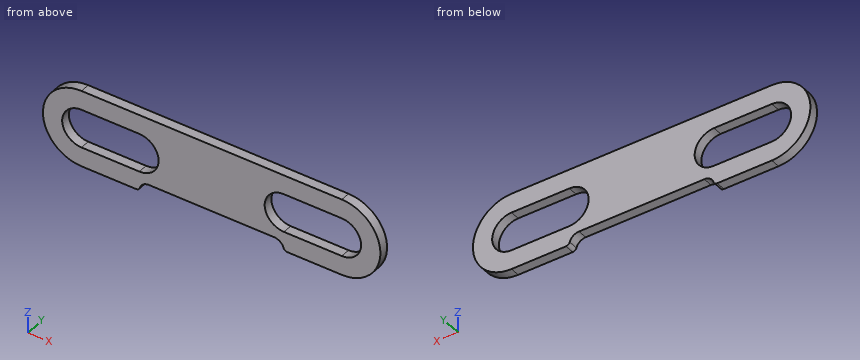
from build123d import *

# Parameters (mm, degrees)
BOSS_EXTRUDE1_DEPTH = 3.175
CUT_EXTRUDE1_DEPTH  = 7.35
FILLET1_R           = 2.54


with BuildPart() as part:
    # Sketch1 → Boss-Extrude1 (new body, symmetric)
    with BuildSketch(Plane(origin=(0, 0, 0), x_dir=(1, 0, 0), z_dir=(0, 1, 0))):
        with BuildLine():
            Line((-85.725, 25.4), (85.725, 25.4))
            ThreePointArc((85.725, 25.4), (111.125, 0), (85.725, -25.4))
            Line((85.725, -25.4), (-85.725, -25.4))
            ThreePointArc((-85.725, -25.4), (-111.125, 0), (-85.725, 25.4))
        make_face()
        with BuildLine():
            Line((-85.725, 12.7), (-47.625, 12.7))
            ThreePointArc((-47.625, 12.7), (-34.925, 0), (-47.625, -12.7))
            Line((-47.625, -12.7), (-85.725, -12.7))
            ThreePointArc((-85.725, -12.7), (-98.425, 0), (-85.725, 12.7))
        make_face(mode=Mode.SUBTRACT)
        with BuildLine():
            Line((85.725, 12.7), (47.625, 12.7))
            ThreePointArc((47.625, 12.7), (34.925, 0), (47.625, -12.7))
            Line((47.625, -12.7), (85.725, -12.7))
            ThreePointArc((85.725, -12.7), (98.425, 0), (85.725, 12.7))
        make_face(mode=Mode.SUBTRACT)
    extrude(amount=BOSS_EXTRUDE1_DEPTH, both=True)

    # Sketch2 → Cut-Extrude1 (cut, through all)
    with BuildSketch(Plane(origin=(0, 3.175, 0), x_dir=(1, 0, 0), z_dir=(0, 1, 0))):
        with BuildLine():
            Line((-41.275, 19.05), (41.275, 19.05))
            ThreePointArc((41.275, 19.05), (45.765128061, 20.909871939), (47.625, 25.4))
            Line((47.625, 25.4), (-47.625, 25.4))
            ThreePointArc((-47.625, 25.4), (-45.765128061, 20.909871939), (-41.275, 19.05))
        make_face()
    extrude(amount=-CUT_EXTRUDE1_DEPTH, mode=Mode.SUBTRACT)

    # Fillet1
    fillet1_edges = [part.edges().sort_by_distance(p)[0] for p in [
        (-47.625, 0, -25.4),
        (47.625, 0, -25.4),
    ]]
    fillet(fillet1_edges, radius=FILLET1_R)


solid = part.part
Model file for the job. Use its own axes, mm. Give positions to 0.01 mm unless a question says otherwise; leave off trailing zeros. Loops run counter-clockwise (first coordinate to the right, second up) from the corner with the lowest first, then second, coordinate; pieces in that order, holes last. Notation, with made-up numbers: (85, -35.75) -> (90, -35.75) arc R33 cw to (90, -3.75) -> close; hole circle Ø3 at (-3.5, 72). An arc over 180 degrees is marked (long way). Use a Markdown table: item, result. Add a question column.
(1) Wall check: line 1 along Z through (x, y) = (63, 0); line 2 along X through (y, z) = (1, 3.5); line 3 along X through (y, z) = (0.5, 1.5). Give the ranges that are in metal, low to high.
(2) Slice it at B-B on z = 0. List the corners of the cut face in (x, y) (3 decimals).
(3) Slice it at C-C on y = -1.25. List the corners of the cut face in (x, z) (3 decimals), and give its area (3 significant figures).
(4) Slice it at D-D on x = -16. List the corners of the cut face in (y, z) (3 decimals), and give its area (3 significant figures).
(5) Drop a flat-ended pin along its axis: pin 1 Ø3 at (y, z) = (-2.5, 3.5) entering from -X. Give the stop position or say it passes through.
(6) Slice it at A-A on x = 57.5. List the corners of the cut face in (y, z) (3 decimals).
Filled sheet:
| question | item | result |
|---|---|---|
| 1 | line 1 | -25.4 to -12.7, 12.7 to 25.4 |
| 1 | line 2 | -110.88 to -97.93, -35.42 to 35.42, 97.93 to 110.88 |
| 1 | line 3 | -111.08 to -98.34, -35.01 to 35.01, 98.34 to 111.08 |
| 2 | outline | (-111.125, -3.175) -> (-98.425, -3.175) -> (-98.425, 3.175) -> (-111.125, 3.175) -> close; (-34.925, -3.175) -> (34.925, -3.175) -> (34.925, 3.175) -> (-34.925, 3.175) -> close; (98.425, -3.175) -> (111.125, -3.175) -> (111.125, 3.175) -> (98.425, 3.175) -> close |
| 3 | outline | (-85.725, -25.4) -> (-49.794, -25.4) arc R2.54 ccw to (-47.36, -23.586) arc R6.35 cw to (-41.275, -19.05) -> (41.275, -19.05) arc R6.35 cw to (47.36, -23.586) arc R2.54 ccw to (49.794, -25.4) -> (85.725, -25.4) arc R25.4 ccw to (85.725, 25.4) -> (-85.725, 25.4) arc R25.4 ccw to start; hole (-85.725, -12.7) -> (-47.625, -12.7) arc R12.7 ccw to (-47.625, 12.7) -> (-85.725, 12.7) arc R12.7 ccw to start; hole (47.625, -12.7) -> (85.725, -12.7) arc R12.7 ccw to (85.725, 12.7) -> (47.625, 12.7) arc R12.7 ccw to start |
| 3 | area | 7,200 mm2 |
| 4 | outline | (-3.175, -19.05) -> (3.175, -19.05) -> (3.175, 25.4) -> (-3.175, 25.4) -> close |
| 4 | area | 282 mm2 |
| 5 | pin 1 | x = -111.05 |
| 6 | outline | (-3.175, -25.4) -> (3.175, -25.4) -> (3.175, -12.7) -> (-3.175, -12.7) -> close; (-3.175, 12.7) -> (3.175, 12.7) -> (3.175, 25.4) -> (-3.175, 25.4) -> close |
